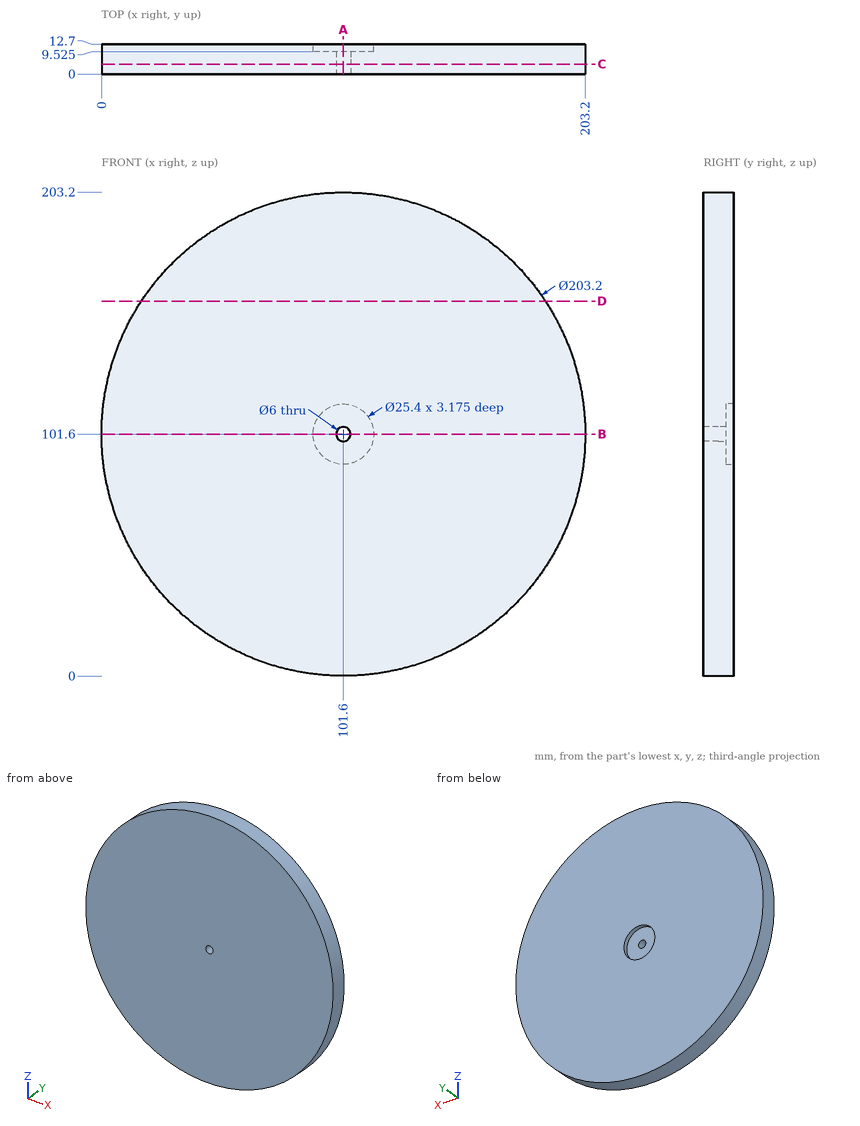
For this review, use the dimensioned drawing (mm, ordinates from the lowest corner) and the shaded views. Round coordinates to 2 decimals unless told otherwise and drop trailing zeros. Write each loop counter-clockwise with the first axis right and the second up, starting at its lowest first coordinate (ties: lowest second). Pieces come first, ordered by that corner, then holes. Notation, with made-up numbers: (73.25, -40) - (124.25, -40) arc R10 cw to (124.25, -32) - close; hole circle Ø6 at (-14, 59.5). An arc over 180 degrees is marked (long way). Answer as a JSON object with one key per item and string values.
1. We need section A-A on x = 101.6. Give the boundary of the cut face in (y, z) (3 decimals), then the cut area to 3 significant figures.
Response values:
{"outline": "(0, 0) - (12.7, 0) - (12.7, 88.9) - (9.525, 88.9) - (9.525, 98.6) - (0, 98.6) - close; (0, 104.6) - (9.525, 104.6) - (9.525, 114.3) - (12.7, 114.3) - (12.7, 203.2) - (0, 203.2) - close", "area": "2,440 mm2"}
2. We need section D-D on z = 157.5. Give the boundary of the cut face in (x, y), then the cut area to 3 significant figures.
Response values:
{"outline": "(16.76, 0) - (186.44, 0) - (186.44, 12.7) - (16.76, 12.7) - close", "area": "2,150 mm2"}
3. For pin 1 Ø1.5 at (x, y) = (83, 10) entering from -Z; pin 2 Ø5 at (x, y) = (69, 7) entering from +Z; pin 3 Ø3 at (y, z) = (4, 63.5) entering from +X, all flat-tipped, find the tip position at first contact; note any pin that passes through.
Response values:
{"pin 1": "stops at z = 1.58", "pin 2": "stops at z = 198.64", "pin 3": "stops at x = 196.38"}
4. We need section C-C on y = 4.25. Give the boundary of the cut face in (x, z).
Response values:
{"outline": "circle Ø203.2 at (101.6, 101.6); hole circle Ø6 at (101.6, 101.6)"}
5. We need section B-B on z = 101.6. Give the boundary of the cut face in (x, y) (3 decimals), then the cut area to 3 significant figures.
Response values:
{"outline": "(0, 0) - (98.6, 0) - (98.6, 9.525) - (88.9, 9.525) - (88.9, 12.7) - (0, 12.7) - close; (104.6, 0) - (203.2, 0) - (203.2, 12.7) - (114.3, 12.7) - (114.3, 9.525) - (104.6, 9.525) - close", "area": "2,440 mm2"}
6. To check wall thickness, follow line 1 along X through (y, z) = (6, 101.6); line 2 along X through (y, z) = (11.2, 101.6); line 3 along X through (y, z) = (6.75, 187). State the ranges of each line that lie inside material, in increasing order.
Response values:
{"line 1": "x = 0 to 98.6, 104.6 to 203.2", "line 2": "x = 0 to 88.9, 114.3 to 203.2", "line 3": "x = 46.56 to 156.64"}
